Verification items for the finished model (mm, model axes). A direction names the side the tool comes from. Give positions to 0.01 mm unless a question says otherwise; leave off trailing zeros. Order: outer loops, then holes, each group sorted by start corner. A loop starts at its lowest first (then second) coordinate and runs counter-clockwise, first axis right, second up. Notation, with made-up numbers: (6, 10.5) -> (64, 10.5) arc R27 ccw to (64, 27.5) -> close; hole circle Ø8 at (-3.5, 54). An arc over 180 degrees is marked (long way). One line per question, with ' | ' between items. Start each with the question number.
Q1. Material ranges on probe 1 along Z at (x, y) = (0, -3); probe 2 along Y at (x, z) = (153.5, 6); probe 3 along Z at (x, y) = (283.5, 26), recorded low to high. Write a range as [from, to].
Q2. Section check C-C on y = -27. Record the cut outline in (x, z), plus the area to 3 significant figures.
Q3. Go/stop test with flat-tipped pins: pin 1 (4 mm diameter, centred on x = 256.5, z = 16.5, fed in from -Y); pin 2 (8 mm diameter, centred on x = 150, z = 5.5, fed in from -Y); pin 3 (2 mm diameter, centred on y = -23.5, z = 20.5, fed in from -X). Record where each tip stops, or that it passes through.
Q4. Section check B-B on x = 277.5. Record the cut outline in (y, z), plus the area to 3 significant figures.
Q5. Mould release check, pull along X, two halves, no side actions. Record for faces 1 (the cylindrical face through (295.975, -7.66, 44.65)), 2 (the flat face through (277, 0, 70)), 3 (the cylindrical face through (-34.97, 1.42, 4.93)): released by +X, released by -X, zero draft, split by the parting line, or undercut.
Q6. Section check A-A on y = 0. Record the cut outline in (x, z), plus the area to 4 significant figures.
Q7. Access from +Z, -Z, +X, -X, +Y, -Y to the whole of each face (thin tool, end or side, straight path). Record for faces 4 (the flat face through (137, 5, 5)), 5 (the flat face through (140.5, 4.7, 0)), 6 (the flat face through (265, 17, 20)), 7 (the flat face through (137, -5, 5)).
Q8. Section check D-D on z = 61. Record the cut outline in (x, y), plus the area to 3 significant figures.
from build123d import *

# Parameters (mm, degrees)
ESBO_O1_R                     = 35
RESSALTO_EXTRUS_O1_DEPTH      = 10
ESBO_O4_W                     = 10
ESBO_O4_H                     = 10
RESSALTO_EXTRUS_O2_DEPTH      = 277.5
FILETE3_R                     = 5
FILETE4_R                     = 5
RESSALTO_EXTRUS_O3_DEPTH      = 10
RESSALTO_EXTRUS_O3_DEPTH_BACK = 10
ESBO_O6_R                     = 35
FILETE5_R                     = 5
FILETE6_R                     = 5
ESBO_O7_R                     = 20
RESSALTO_EXTRUS_O4_DEPTH      = 50


with BuildPart() as part:
    # Esboço1 → Ressalto-extrusão1 (new body)
    with BuildSketch(Plane(origin=(0, 0, 0), x_dir=(0, 1, 0), z_dir=(0, 0, 1))):
        with Locations(Location((0, 0, 0), (0, 0, 270))):
            Circle(ESBO_O1_R)
    extrude(amount=RESSALTO_EXTRUS_O1_DEPTH)

    # Esboço4 → Ressalto-extrusão2 (add)
    with BuildSketch(Plane.YZ):
        with Locations((0, 5)):
            Rectangle(ESBO_O4_W, ESBO_O4_H)
    extrude(amount=RESSALTO_EXTRUS_O2_DEPTH)

    # Filete3
    filete3_edges = [part.edges().sort_by_distance(p)[0] for p in [
        (34.641016151, -5, 5),
    ]]
    fillet(filete3_edges, radius=FILETE3_R)

    # Filete4
    filete4_edges = [part.edges().sort_by_distance(p)[0] for p in [
        (34.641016151, 5, 5),
    ]]
    fillet(filete4_edges, radius=FILETE4_R)

    # Esboço6 → Ressalto-extrusão3 (add, two sides: drawn at the far end of the back side and taken through both)
    with BuildSketch(Plane.XY.offset(10).offset(-RESSALTO_EXTRUS_O3_DEPTH_BACK)):
        with Locations(Location((277.5, 0, 0), (0, 0, 171.786789298))):
            Circle(ESBO_O6_R)
    extrude(amount=RESSALTO_EXTRUS_O3_DEPTH + RESSALTO_EXTRUS_O3_DEPTH_BACK)

    # Filete5
    filete5_edges = [part.edges().sort_by_distance(p)[0] for p in [
        (242.858983849, -5, 5),
    ]]
    fillet(filete5_edges, radius=FILETE5_R)

    # Filete6
    # the kernel refuses this fillet: 5 mm, written as the material it adds along each edge
    with BuildSketch(Plane(origin=(242.858983849, 5, 10), x_dir=(0.1967224418008006, 0.9804592193925918, 0), z_dir=(0, 0, -1))) as filete6_piece_1:
        with BuildLine():
            CenterArc((4.097933971, -4.992530838), FILETE6_R, 93.132150742, 75.522487814)
            Line((-0.804362126, -4.008918629), (0, 0))
            ThreePointArc((0, 0), (1.912369187, -0.052284136), (3.824738373, 0))
        make_face()
    extrude(amount=10)

    # Esboço7 → Ressalto-extrusão4 (add)
    with BuildSketch(Plane.XY.offset(20)):
        with Locations((277.5, 0)):
            Circle(ESBO_O7_R)
    extrude(amount=RESSALTO_EXTRUS_O4_DEPTH)


solid = part.part
Filled in:
1) probe 1: [0, 10] | probe 2: [-5, 5] | probe 3: [0, 20]
2) outline: (-22.27, 0) -> (22.27, 0) -> (22.27, 10) -> (-22.27, 10) -> close; (255.23, 0) -> (299.77, 0) -> (299.77, 20) -> (255.23, 20) -> close | area: 1,340 mm²
3) pin 1: y = -29.39 | pin 2: y = -5 | pin 3: x = 250.8
4) outline: (-35, 0) -> (35, 0) -> (35, 20) -> (20, 20) -> (20, 70) -> (-20, 70) -> (-20, 20) -> (-35, 20) -> close | area: 3,400 mm²
5) face 1: split by the parting line | face 2: zero draft | face 3: undercut
6) outline: (-35, 0) -> (312.5, 0) -> (312.5, 20) -> (297.5, 20) -> (297.5, 70) -> (257.5, 70) -> (257.5, 20) -> (242.5, 20) -> (242.5, 10) -> (-35, 10) -> close | area: 6,175 mm²
7) face 4: +Z, -Z, +Y | face 5: -Z, +X, -X, +Y, -Y | face 6: +Z | face 7: +Z, -Z, -Y
8) outline: circle Ø40 at (277.5, 0) | area: 1,260 mm²
